Check sheet for the modelled part. Datum: model origin and axes. Units: mm. A direction names the side the tool comes from. Coordinates: 2 decimals unless noted, no trailing zeros. Loops run counter-clockwise (first coordinate to the right, second up) from the corner with the lowest first, then second, coordinate; pieces in that order, holes last. Notation, with made-up numbers: M 59,10.5 L 78,10.5 A19 cw 78,37.5 Z; hole C 66.25,53.5 d2. An arc over 180 degrees is marked long. Return JSON: item names as keys, results as strings.
from build123d import *

# Parameters (mm, degrees)
BOSS_EXTRUDE1_DEPTH                     = 6.35
SKETCH4_W                               = 40
SKETCH4_H                               = 35
CUT_EXTRUDE1_DEPTH                      = 135.686014493
FILLET1_R                               = 5
CBORE_FOR_M5_HEX_HEAD_BOLT1_D           = 5.8
CBORE_FOR_M5_HEX_HEAD_BOLT1_CBORE_D     = 12.24
CBORE_FOR_M5_HEX_HEAD_BOLT1_CBORE_DEPTH = 3.58
FILLET2_R                               = 10
FILLET3_R                               = 2
CBORE_FOR_M3_SHCS1_D                    = 3.4
CBORE_FOR_M3_SHCS1_CBORE_D              = 6.5
CBORE_FOR_M3_SHCS1_CBORE_DEPTH          = 3
M5X0_8_TAPPED_HOLE1_D                   = 4.2


with BuildPart() as part:
    # Sketch1 → Boss-Extrude1 (new body)
    with BuildSketch(Plane(origin=(0, 0, 0), x_dir=(1, 0, 0), z_dir=(0, 1, 0))):
        Polygon((55, -55), (-55, -55), (-55, -17.5), (-100, -17.5), (-100, 17.5), (-55, 17.5), (-90, 55), (-90, 90), (-55, 90), (-55, 55), (-17.5, 55), (-17.5, 90), (17.5, 90), (17.5, 55), (55, 55), (55, 90), (90, 90), (90, 55), (55, 17.5), (100, 17.5), (100, -17.5), (55, -17.5), align=None)
    extrude(amount=BOSS_EXTRUDE1_DEPTH)

    # Sketch4 → Cut-Extrude1 (cut, through all)
    with BuildSketch(Plane(origin=(0, 6.35, 0), x_dir=(1, 0, 0), z_dir=(0, 1, 0))):
        with Locations((0, -37.5)):
            Rectangle(SKETCH4_W, SKETCH4_H)
    extrude(amount=-CUT_EXTRUDE1_DEPTH, mode=Mode.SUBTRACT)

    # Fillet1
    fillet1_edges = [part.edges().sort_by_distance(p)[0] for p in [
        (-90, 3.175, -55),
        (-90, 3.175, -90),
        (-55, 3.175, -90),
        (-55, 3.175, -55),
        (-17.5, 3.175, -55),
        (-17.5, 3.175, -90),
        (17.5, 3.175, -90),
        (17.5, 3.175, -55),
        (55, 3.175, -55),
        (55, 3.175, -90),
        (90, 3.175, -90),
        (90, 3.175, -55),
        (55, 3.175, -17.5),
        (100, 3.175, -17.5),
        (100, 3.175, 17.5),
        (55, 3.175, 17.5),
        (55, 3.175, 55),
        (-55, 3.175, 55),
        (-55, 3.175, 17.5),
        (-100, 3.175, 17.5),
        (-100, 3.175, -17.5),
        (-55, 3.175, -17.5),
        (20, 3.175, 55),
        (-20, 3.175, 55),
    ]]
    fillet(fillet1_edges, radius=FILLET1_R)

    # CBORE for M5 Hex Head Bolt1 (through all)
    with Locations(Plane.XZ):
        with Locations((-45, 45), (-45, -45), (45, -45), (45, 45)):
            CounterBoreHole(CBORE_FOR_M5_HEX_HEAD_BOLT1_D / 2, CBORE_FOR_M5_HEX_HEAD_BOLT1_CBORE_D / 2, CBORE_FOR_M5_HEX_HEAD_BOLT1_CBORE_DEPTH)

    # Fillet2
    fillet2_edges = [part.edges().sort_by_distance(p)[0] for p in [
        (-20, 3.175, 20),
        (20, 3.175, 20),
    ]]
    fillet(fillet2_edges, radius=FILLET2_R)

    # Fillet3
    # the kernel refuses this fillet: 2 mm, written as the material it takes off along each edge
    with BuildSketch(Plane(origin=(20, 6.35, 30), x_dir=(0, -1, 0), z_dir=(0, 0, 1)), Plane(origin=(-20, 6.35, 55), x_dir=(0, -1, 0), z_dir=(0, 0, -1))) as fillet3_piece_1:
        with BuildLine():
            CenterArc((FILLET3_R, FILLET3_R), FILLET3_R, 180, 90)
            Line((0, FILLET3_R), (0, 0))
            Line((0, 0), (FILLET3_R, 0))
        make_face()
    extrude(amount=25, mode=Mode.SUBTRACT)
    with BuildSketch(Plane(origin=(-10, 6.35, 20), x_dir=(0, -1, 0), z_dir=(1, 0, 0))) as fillet3_piece_2:
        with BuildLine():
            CenterArc((FILLET3_R, FILLET3_R), FILLET3_R, 180, 90)
            Line((0, FILLET3_R), (0, 0))
            Line((0, 0), (FILLET3_R, 0))
        make_face()
    extrude(amount=20, mode=Mode.SUBTRACT)
    with BuildSketch(Plane(origin=(-20, 0, 30), x_dir=(-1, 0, 0), z_dir=(0, 0, 1)), Plane(origin=(20, 0, 55), x_dir=(1, 0, 0), z_dir=(0, 0, -1))) as fillet3_piece_3:
        with BuildLine():
            CenterArc((FILLET3_R, -FILLET3_R), FILLET3_R, 90, 90)
            Line((0, -FILLET3_R), (0, 0))
            Line((0, 0), (FILLET3_R, 0))
        make_face()
    extrude(amount=25, mode=Mode.SUBTRACT)
    with BuildSketch(Plane(origin=(10, 0, 20), x_dir=(0, 0, -1), z_dir=(-1, 0, 0))) as fillet3_piece_4:
        with BuildLine():
            CenterArc((FILLET3_R, -FILLET3_R), FILLET3_R, 90, 90)
            Line((0, -FILLET3_R), (0, 0))
            Line((0, 0), (FILLET3_R, 0))
        make_face()
    extrude(amount=20, mode=Mode.SUBTRACT)
    with BuildSketch(Plane(origin=(10, 0, 30), x_dir=(1, 0, 0), z_dir=(0, 0, 1))) as fillet3_piece_5:
        with BuildLine():
            CenterArc((10 + FILLET3_R, FILLET3_R), FILLET3_R, 180, 90)
            Line((10, FILLET3_R), (10, 0))
            Line((10, 0), (10 + FILLET3_R, 0))
        make_face()
    revolve(axis=Axis((10, 0, 30), (0, 1, 0)), revolution_arc=90, mode=Mode.SUBTRACT)
    with BuildSketch(Plane(origin=(-10, 0, 30), x_dir=(0, 0, -1), z_dir=(1, 0, 0))) as fillet3_piece_6:
        with BuildLine():
            CenterArc((10 + FILLET3_R, FILLET3_R), FILLET3_R, 180, 90)
            Line((10, FILLET3_R), (10, 0))
            Line((10, 0), (10 + FILLET3_R, 0))
        make_face()
    revolve(axis=Axis((-10, 0, 30), (0, 1, 0)), revolution_arc=90, mode=Mode.SUBTRACT)
    with BuildSketch(Plane(origin=(-10, 6.35, 30), x_dir=(0, 0, -1), z_dir=(1, 0, 0))) as fillet3_piece_7:
        with BuildLine():
            CenterArc((10 + FILLET3_R, -FILLET3_R), FILLET3_R, 90, 90)
            Line((10 + FILLET3_R, 0), (10, 0))
            Line((10, 0), (10, -FILLET3_R))
        make_face()
    revolve(axis=Axis((-10, 6.35, 30), (0, 1, 0)), revolution_arc=90, mode=Mode.SUBTRACT)
    with BuildSketch(Plane(origin=(10, 6.35, 30), x_dir=(1, 0, 0), z_dir=(0, 0, 1))) as fillet3_piece_8:
        with BuildLine():
            CenterArc((10 + FILLET3_R, -FILLET3_R), FILLET3_R, 90, 90)
            Line((10 + FILLET3_R, 0), (10, 0))
            Line((10, 0), (10, -FILLET3_R))
        make_face()
    revolve(axis=Axis((10, 6.35, 30), (0, 1, 0)), revolution_arc=90, mode=Mode.SUBTRACT)

    # CBORE for M3 SHCS1 (through all)
    with Locations(Plane(origin=(0, 0, 0), x_dir=(-1, 0, 0), z_dir=(0, -1, 0))):
        with Locations((10, 84), (-10, 84), (0, 60.3), (-94, 10), (-94, -10), (-70.3, 0), (94, -10), (94, 10), (70.3, 0), (-82.5, 84), (-62.5, 84), (-72.5, 60.3), (72.5, 60.3), (82.5, 84), (62.5, 84)):
            CounterBoreHole(CBORE_FOR_M3_SHCS1_D / 2, CBORE_FOR_M3_SHCS1_CBORE_D / 2, CBORE_FOR_M3_SHCS1_CBORE_DEPTH)

    # M5x0.8 Tapped Hole1 (through all)
    with Locations(Plane(origin=(0, 0, 0), x_dir=(-1, 0, 0), z_dir=(0, -1, 0))):
        with Locations((-20, 15), (20, 15), (20, -5), (-20, -5), (-30, 15), (-30, -5), (30, 15), (30, -5)):
            Hole(M5X0_8_TAPPED_HOLE1_D / 2)


solid = part.part
1) Go/stop test with flat-tipped pins: pin 1 Ø3 at (y, z) = (1.5, -57) entering from -X; pin 2 Ø3 at (y, z) = (4, -27.5) entering from +X; pin 3 Ø1.5 at (y, z) = (2.5, -36.5) entering from +X. Record where each tip stops, or that it passes through.
Answers:
{"pin 1": "x = -90", "pin 2": "x = 65.73", "pin 3": "x = 73.43"}
2) Section check A-A on z = -73.5. Record the cut outline in (x, y), then the cut area to 3 significant figures.
Answers:
{"outline": "M -90,0 L -55,0 L -55,6.35 L -90,6.35 Z; M -17.5,0 L 17.5,0 L 17.5,6.35 L -17.5,6.35 Z; M 55,0 L 90,0 L 90,6.35 L 55,6.35 Z", "area": "667 mm²"}
3) Set-up check for faces 4 (the face through (75.079, 1.479, -58.322)), 5 (the face through (-100, 3, 0)), 6 (the face through (-56, 3, -88)): record each of +Z, -Z, +X, -X, +Y, -Y from which the full face is reachable in a straight line by a thin tool's end or side.
Answers:
{"face 4": "-Y", "face 5": "+Z, -Z, -X, +Y, -Y", "face 6": "-Z, +Y, -Y"}
4) Section check C-C on z = -45. Record the cut outline in (x, y), then the cut area to 3 significant figures.
Answers:
{"outline": "M -80.67,0 L -51.12,0 L -51.12,3.58 L -47.9,3.58 L -47.9,6.35 L -80.67,6.35 Z; M -42.1,3.58 L -38.88,3.58 L -38.88,0 L 38.88,0 L 38.88,3.58 L 42.1,3.58 L 42.1,6.35 L -42.1,6.35 Z; M 47.9,3.58 L 51.12,3.58 L 51.12,0 L 80.67,0 L 80.67,6.35 L 47.9,6.35 Z", "area": "905 mm²"}
5) Section check B-B on x = -30. Record the cut outline in (y, z).
Answers:
{"outline": "M 0,-55 L 6.35,-55 L 6.35,-17.1 L 0,-17.1 Z; M 0,-12.9 L 6.35,-12.9 L 6.35,2.9 L 0,2.9 Z; M 0,7.1 L 6.35,7.1 L 6.35,55 L 0,55 Z"}
6) Draft check along X on faces 1 (the face through (-55, 3, 36)), 2 (the face through (63.205, 1.479, -80.827)), 3 (the face through (61.953, 3.219, -20.433)). Enter one of: +X half, -X half, draft (parallel to the pull), parting line (faces both ways), or undercut.
Answers:
{"face 1": "-X half", "face 2": "undercut", "face 3": "+X half"}
7) Scan lines: line 1 along Z through (x, y) = (94, 1.25); line 2 along Z through (x, y) = (30, 2.75); line 3 along X through (y, z) = (3.5, 4.5). Record each from-to range of solid material in increasing order. Write a range as [from, to].
Answers:
{"line 1": "[-17.5, -13.25], [-6.75, 6.75], [13.25, 17.5]", "line 2": "[-55, -17.1], [-12.9, 2.9], [7.1, 55]", "line 3": "[-100, -32.04], [-27.96, -22.04], [-17.96, 17.96], [22.04, 27.96], [32.04, 100]"}
